Verification items for the finished model (mm, model axes). Give positions to 0.01 mm unless a question says otherwise; leave off trailing zeros. Answer as a JSON object with one key per item and string values. Group by question number.
Item 1: Sectioned sample at A-A, the plane z = 0.65. Count the separate pieces of the cut face and the enclosed holes in it, and give its area (3 significant figures).
Item 2: Go/stop test with flat-tipped pins: pin 1 (2 mm diameter, centred on y = -16, z = 2.5, fed in from -X); pin 2 (1.2 mm diameter, centred on x = 107, z = 2, fed in from -Y); pin 3 (1.5 mm diameter, centred on x = -44, z = 1.5, fed in from -Y). Record where each tip stops, or that it passes through.
Item 3: Scan lines: line 1 along X through (y, z) = (-44, 2.9); line 2 along X through (y, z) = (-15.5, 0.2); line 3 along X through (y, z) = (-18, 1). Record each from-to range of solid material in increasing order. Write a range as [from, to].
```python
from build123d import *

# Parameters (mm, degrees)
SKETCH1_R           = 11
BOSS_EXTRUDE1_DEPTH = 4
SKETCH2_R           = 1.5
CUT_EXTRUDE1_DEPTH  = 10
CUT_EXTRUDE2_START  = -10
CUT_EXTRUDE2_DEPTH  = 10
FILLET1_R           = 10
FILLET3_R           = 3
SKETCH5_W           = 30
SKETCH5_H           = 5
CUT_EXTRUDE4_DEPTH  = 10
SKETCH6_R           = 2.5
CUT_EXTRUDE5_DEPTH  = 177.821944339
SKETCH8_R           = 2
CUT_EXTRUDE7_DEPTH  = 177.821944339


with BuildPart() as part:
    # Sketch1 → Boss-Extrude1 (new body)
    with BuildSketch(Plane.XY):
        with BuildLine():
            Line((-115.233797414, -48.437298991), (-115.233797414, -6.093952298))
            Line((-115.233797414, -6.093952298), (-83.233797414, -6.093952298))
            Line((-83.233797414, -6.093952298), (-83.233797414, -93.258431083))
            ThreePointArc((-83.233797414, -93.258431083), (0, -125), (83.233797414, -93.258431083))
            Line((83.233797414, -93.258431083), (83.233797414, -6.093952298))
            Line((83.233797414, -6.093952298), (115.233797414, -6.093952298))
            Line((115.233797414, -6.093952298), (115.233797414, -48.437298991))
            ThreePointArc((115.233797414, -48.437298991), (0, 125), (-115.233797414, -48.437298991))
        make_face()
        with Locations((0, 80)):
            Circle(SKETCH1_R, mode=Mode.SUBTRACT)
    extrude(amount=BOSS_EXTRUDE1_DEPTH)

    # Sketch2 → Cut-Extrude1 (cut)
    with BuildSketch(Plane.XY.offset(4)):
        with Locations((0, 92.990381057)):
            Circle(SKETCH2_R)
        with Locations((11.25, 73.504809472)):
            Circle(SKETCH2_R)
        with Locations((-11.25, 73.504809472)):
            Circle(SKETCH2_R)
    extrude(amount=-CUT_EXTRUDE1_DEPTH, mode=Mode.SUBTRACT)

    # Sketch3 → Cut-Extrude2 (cut)
    with BuildSketch(Plane.XY.offset(4).offset(CUT_EXTRUDE2_START)):
        with BuildLine():
            Line((-83.233797414, -93.258431083), (83.233797414, -93.258431083))
            ThreePointArc((83.233797414, -93.258431083), (0, -125), (-83.233797414, -93.258431083))
        make_face()
    extrude(amount=CUT_EXTRUDE2_DEPTH, mode=Mode.SUBTRACT)

    # Fillet1
    fillet1_edges = [part.edges().sort_by_distance(p)[0] for p in [
        (83.233797414, -93.258431083, 2),
        (-83.233797414, -93.258431083, 2),
    ]]
    fillet(fillet1_edges, radius=FILLET1_R)

    # Fillet3
    fillet3_edges = [part.edges().sort_by_distance(p)[0] for p in [
        (115.233797414, -48.437298991, 2),
        (-115.233797414, -48.437298991, 2),
    ]]
    fillet(fillet3_edges, radius=FILLET3_R)

    # Sketch5 → Cut-Extrude4 (cut)
    with BuildSketch(Plane.XY.offset(4)):
        with Locations((38.233797414, -90.758431083)):
            Rectangle(SKETCH5_W, SKETCH5_H)
        with Locations((-38.233797414, -90.758431083)):
            Rectangle(SKETCH5_W, SKETCH5_H)
    extrude(amount=-CUT_EXTRUDE4_DEPTH, mode=Mode.SUBTRACT)

    # Sketch6 → Cut-Extrude5 (cut, through all)
    with BuildSketch(Plane.XY.offset(4)):
        with Locations((-73.5, -82.645466924)):
            Circle(SKETCH6_R)
        with Locations((73.5, -82.645466924)):
            Circle(SKETCH6_R)
        with Locations((73.5, 27.354533076)):
            Circle(SKETCH6_R)
        with Locations((-73.5, 27.354533076)):
            Circle(SKETCH6_R)
    extrude(amount=-CUT_EXTRUDE5_DEPTH, mode=Mode.SUBTRACT)

    # Sketch8 → Cut-Extrude7 (cut, through all)
    with BuildSketch(Plane.XY.offset(4)):
        with Locations((46.115537646, -27.497588789)):
            Circle(SKETCH8_R)
        with Locations((46.115537646, -44.497588789)):
            Circle(SKETCH8_R)
        with Locations((60.115537646, -44.497588789)):
            Circle(SKETCH8_R)
        with Locations((60.115537646, -27.497588789)):
            Circle(SKETCH8_R)
    cut_extrude7 = extrude(amount=-CUT_EXTRUDE7_DEPTH, mode=Mode.SUBTRACT)

    # Mirror2: Cut-Extrude7 across plane
    add(cut_extrude7.mirror(Plane.ZY), mode=Mode.SUBTRACT)


solid = part.part
```
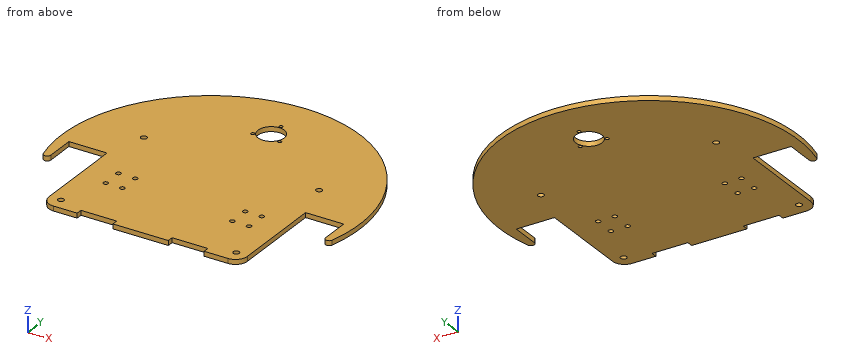
Geometry check:
{
 "1": {"separate pieces": "1", "enclosed holes": "16", "area": "40,100 mm^2"},
 "2": {"pin 1": "x = -124.1", "pin 2": "y = -6.09", "pin 3": "y = -88.26"},
 "3": {"line 1": "[-83.23, -62.05], [-58.18, -48.05], [-44.18, 44.18], [48.05, 58.18], [62.05, 83.23]", "line 2": "[-124.04, -115.23], [-83.23, 83.23], [115.23, 124.04]", "line 3": "[-123.7, -115.23], [-83.23, 83.23], [115.23, 123.7]"}
}
